Model file for the job. Use its own axes, mm. A direction names the side the tool comes from. Give positions to 0.01 mm unless a question says otherwise; leave off trailing zeros. Loops run counter-clockwise (first coordinate to the right, second up) from the corner with the lowest first, then second, coordinate; pieces in that order, holes last. Notation, with made-up numbers: M -25.5,18.5 L 3.5,18.5 A14 cw 3.5,37.5 Z; hole C -29,28 d8. An arc over 180 degrees is marked long. Answer in a Markdown table with one row per item.
```python
from build123d import *

# Parameters (mm, degrees)
F0_R     = 1.115605
F0_R_2   = 1.412634
F1_DEPTH = 3
F2_DEPTH = 2
F3_DEPTH = 1


with BuildPart() as f1:
    # F0 (on Front) → F1 (new body)
    with BuildSketch(Plane.XZ):
        with BuildLine():
            Line((-18.974544, 5.53028), (-18.974544, 3.961724))
            Line((-18.974544, 3.961724), (-18.974544, -4.449865))
            ThreePointArc((-18.974544, -4.449865), (-16.691878, -8.113439), (-16.490631, -12.425264))
            ThreePointArc((-16.490631, -12.425264), (-14.938687, -12.937181), (-13.308015, -13.044414))
            ThreePointArc((-13.308015, -13.044414), (-9.397709, -13.283603), (-5.487403, -13.044414))
            ThreePointArc((-5.487403, -13.044414), (-4.138982, -13.179799), (-2.879113, -12.680498))
            ThreePointArc((-2.879113, -12.680498), (-4.33521, -7.817834), (-1.669094, -3.498396))
            Line((-1.669094, -3.498396), (-1.669094, 5.53028))
            Line((-1.669094, 5.53028), (-6.735639, 0))
            ThreePointArc((-6.735639, 0), (-10.548048, 0.838268), (-14.360456, 0))
            Line((-14.360456, 0), (-18.974544, 5.53028))
        make_face()
        Polygon((-10.116423, -11.184998), (-11.513611, -8.5759), (-9.122775, -8.573417), align=None, mode=Mode.SUBTRACT)
        with Locations((-12.903409, -3.036485)):
            Circle(F0_R, mode=Mode.SUBTRACT)
        with Locations((-8.460215, -3.036485)):
            Circle(F0_R_2, mode=Mode.SUBTRACT)
    extrude(amount=F1_DEPTH)

    # F0 (on Front) → F2 (join)
    with BuildSketch(Plane.XZ):
        with BuildLine():
            ThreePointArc((-16.490631, -12.425264), (-16.691878, -8.113439), (-18.974544, -4.449865))
            Line((-18.974544, -4.449865), (-18.974544, -10.341382))
            ThreePointArc((-18.974544, -10.341382), (-17.865075, -11.541243), (-16.490631, -12.425264))
        make_face()
        with BuildLine():
            ThreePointArc((-1.669094, -3.498396), (-4.33521, -7.817834), (-2.879113, -12.680498))
            ThreePointArc((-2.879113, -12.680498), (-1.989511, -11.658159), (-1.669094, -10.341382))
            Line((-1.669094, -10.341382), (-1.669094, -3.498396))
        make_face()
    extrude(amount=F2_DEPTH)

    # F0 (on Front) → F3 (join)
    with BuildSketch(Plane.XZ):
        Polygon((-9.122775, -8.573417), (-11.513611, -8.5759), (-10.116423, -11.184998), align=None)
    extrude(amount=F3_DEPTH)


solid = f1.part
```
Q1. Saw through at B-B (y = -0.5). Give the cut face in (x, z) (1 decimal), and give its area (3 significant figures).
Reported:
| item | result |
|---|---|
| outline | M -19,-10.3 A6.5 ccw -16.5,-12.4 A6.5 ccw -13.3,-13 A32.1 ccw -5.5,-13 A2.9 ccw -2.9,-12.7 A2.9 ccw -1.7,-10.3 L -1.7,5.5 L -6.7,0 A9.1 ccw -14.4,0 L -19,5.5 Z; hole C -12.9,-3 d2.2; hole C -8.5,-3 d2.8 |
| area | 242 mm² |
Q2. Saw through at A-A (x = -8). Give the cut face in (y, z), and give its area (3 significant figures).
Reported:
| item | result |
|---|---|
| outline | M -3,-13.25 L 0,-13.25 L 0,-4.37 L -3,-4.37 Z; M -3,-1.7 L 0,-1.7 L 0,0.47 L -3,0.47 Z |
| area | 33.2 mm² |
Q3. Saw through at C-C (y = -2.3). Give the cut face in (x, z) (1 decimal).
Reported:
| item | result |
|---|---|
| outline | M -19,-4.4 A8.5 cw -16.5,-12.4 A6.5 ccw -13.3,-13 A32.1 ccw -5.5,-13 A2.9 ccw -2.9,-12.7 A6.2 cw -1.7,-3.5 L -1.7,5.5 L -6.7,0 A9.1 ccw -14.4,0 L -19,5.5 Z; hole C -12.9,-3 d2.2; hole M -11.5,-8.6 L -10.1,-11.2 L -9.1,-8.6 Z; hole C -8.5,-3 d2.8 |
Q4. Probe probe 1 along Z at (x, y) = (-7.5, -0.35); probe 2 along Z at (x, y) = (-8.5, -0.3); probe 3 along X at (y, z) = (-2.3, 1.5). List the from-to ranges inside material, lowest first.
Reported:
| item | result |
|---|---|
| probe 1 | -13.23 to -4.07, -2 to 0.31 |
| probe 2 | -13.27 to -4.45, -1.62 to 0.6 |
| probe 3 | -18.97 to -15.61, -5.36 to -1.67 |
Q5. 3-axis set-ups, long thin cutter, end or side, ignore diameter. For faces 5 (the face through (-16.64, -1.48, 2.73)), 6 (the face through (-3, -2, -8)), 7 (the face through (-16.71, -2.49, -8.06)), 8 (the face through (-10, -1, -10)): which of +Z, -Z, +X, -X, +Y, -Y reach the whole face in a straight line?
Reported:
| item | result |
|---|---|
| face 5 | +Z, +Y, -Y |
| face 6 | +X, -Y |
| face 7 | -X, -Y |
| face 8 | -Y |
Q6. Mould opens along X. For faces 1 (the face through (-7.113, -1.479, -2.612)), 2 (the face through (-4.17, -1.48, 2.8)), 3 (the face through (-1.669, -1, -3)), 4 (the face through (-18, -2, -8)) say: released by +X, released by -X, zero draft, split by the parting line, or undercut.
Reported:
| item | result |
|---|---|
| face 1 | undercut |
| face 2 | undercut |
| face 3 | released by +X |
| face 4 | zero draft |
Q7. Saw through at D-D (x = -4). Give the cut face in (y, z).
Reported:
| item | result |
|---|---|
| outline | M -3,-13.16 L 0,-13.16 L 0,2.99 L -3,2.99 L -3,-6.47 L -2,-6.47 L -2,-10.79 L -3,-10.79 Z |
Q8. Drop a flat-ended pin along its axis: pin 1 (2 mm diameter, centred on x = -18, z = -8.5, fed in from -Y). Give the stop position or say it passes through.
Reported:
| item | result |
|---|---|
| pin 1 | y = -2 |
